Here's how the part is built. I have some questions about the finished solid (model axes, mm). A direction names the side the tool comes from. Coordinates: 2 decimals unless noted, no trailing zeros. Loops run counter-clockwise (first coordinate to the right, second up) from the corner with the lowest first, then second, coordinate; pieces in that order, holes last. Notation, with made-up numbers: M 78,65.25 L 112,65.25 A22 cw 112,86.25 Z; hole C -27.75,-1.5 d4. An arc over 180 degrees is marked long. Use CSV: the item, a comma, the result in double quotes. Start each with the question number.
Q1. Which directions (+Z, -Z, +X, -X, +Y, -Y) give clear straight access to the entire face, cutting with the end or side of a thin tool? Please do faces 1 (the flat face through (1, 0, -5)), 2 (the flat face through (1.49, 2, -5.23)), 3 (the flat face through (1.49, -2, -5.23)), 4 (the cylindrical face through (2.5, 0, -2.5)), 5 (the cylindrical face through (-1.08, -4.88, 24.65)).
Q2. If we section it at D-D (y = 3): Please give me the cut outline in (x, z), and give its area (3 significant figures).
Q3. If we mould it in two halves opening along Z, with no side actions, what happens to faces 6 (the cylindrical face through (-2.5, 0, -2.5)), 7 (the flat face through (-1.47, -2, -5.23)), 8 (the flat face through (0, 0, 50))? For each: +Z half, -Z half, draft (parallel to the pull), parting line (faces both ways), or undercut.
Q4. If we section it at C-C (x = 0): Please give me the cut outline in (y, z).
Q5. If we section it at A-A (y = 0): Please give me the cut outline in (x, z).
Q6. If we section it at B-B (z = 27): Please give me the cut outline in (x, y).
Q7. Please list where these lines run through material, in increasing order: probe 1 along Z at (x, y) = (0.75, 0.25); probe 2 along X at (y, z) = (-4, 32); probe 3 along X at (y, z) = (3.75, 23.5). Write a range as [from, to].
Q8. For pin 1 Ø2 at (y, z) = (0, -6) entering from -X; pin 2 Ø3 at (y, z) = (-1, -7) entering from +X; pin 3 Ø0.6 at (x, z) = (-1.5, -3.5) entering from -Y, each with a flat end and sliding along its axis, tell me the tip position at first contact or that it passes through.
from build123d import *

# Parameters (mm, degrees)
SKETCH1_R           = 5
BOSS_EXTRUDE1_DEPTH = 50
SKETCH4_R           = 2.5
BOSS_EXTRUDE3_DEPTH = 5
SKETCH10_W          = 2
SKETCH10_H          = 10.578661844
CUT_EXTRUDE4_DEPTH  = 51.497524692
SKETCH11_W          = 10
SKETCH11_H          = 0.828427125
CUT_EXTRUDE5_DEPTH  = 51.497524692


with BuildPart() as part:
    # Sketch1 → Boss-Extrude1 (new body)
    with BuildSketch(Plane.XY):
        Circle(SKETCH1_R)
    extrude(amount=BOSS_EXTRUDE1_DEPTH)

    # Sketch4 → Boss-Extrude3 (add)
    with BuildSketch(Plane(origin=(0, 0, 0), x_dir=(-1, 0, 0), z_dir=(0, 0, -1))):
        Circle(SKETCH4_R)
    extrude(amount=BOSS_EXTRUDE3_DEPTH)

    # Sketch8 → Revolve1 (revolve)
    with BuildSketch(Plane(origin=(0, 0, 0), x_dir=(0, 0, -1), z_dir=(1, 0, 0))):
        with BuildLine():
            Line((6.658312395, 3), (6.658312395, -3))
            ThreePointArc((6.658312395, -3), (3.658312395, 0), (6.658312395, 3))
        make_face()
    revolve(axis=Axis((0, 3, -6.658312395), (0, -1, 0)))

    # Sketch10 → Cut-Extrude4 (cut, through all)
    with BuildSketch(Plane(origin=(0, 0, 0), x_dir=(-1, 0, 0), z_dir=(0, 0, -1))):
        Rectangle(SKETCH10_W, SKETCH10_H)
    extrude(amount=CUT_EXTRUDE4_DEPTH, mode=Mode.SUBTRACT)

    # Sketch11 → Cut-Extrude5 (cut, through all)
    with BuildSketch(Plane(origin=(0, 0, 0), x_dir=(-1, 0, 0), z_dir=(0, 0, -1))):
        with Locations((0, 2.414213563)):
            Rectangle(SKETCH11_W, SKETCH11_H)
        with Locations((0, -2.414213563)):
            Rectangle(SKETCH11_W, SKETCH11_H)
    extrude(amount=CUT_EXTRUDE5_DEPTH, mode=Mode.SUBTRACT)


solid = part.part
Results below:
1,face 1,"-Z, +Y, -Y"
1,face 2,"-Z, +X, -X, +Y"
1,face 3,"-Z, +X, -X, -Y"
1,face 4,"+X"
1,face 5,"+Z, -Z"
2,outline,"M -4,0 L 4,0 L 4,50 L -4,50 Z"
2,area,"400 mm^2"
3,face 6,"undercut"
3,face 7,"draft"
3,face 8,"+Z half"
4,outline,"M -5,0 L 5,0 L 5,50 L -5,50 Z"
5,outline,"M -5,0 L -2.5,0 L -2.5,-5 A3 ccw -1,-9.49 L -1,0 L 1,0 L 1,-9.49 A3 ccw 2.5,-5 L 2.5,0 L 5,0 L 5,50 L -5,50 Z"
6,outline,"C 0,0 d10"
7,probe 1,"[0, 50]"
7,probe 2,"[-3, 3]"
7,probe 3,"[-3.31, 3.31]"
8,pin 1,"x = -3"
8,pin 2,"x = 3"
8,pin 3,"y = -2"
